The listing builds one solid part. Answer for the finished solid, in the listing's coordinates (mm). Coordinates: 2 decimals unless noted, no trailing zeros. Write each loop counter-clockwise with the first axis right and the second up, starting at its lowest first coordinate (ties: lowest second). Pieces come first, ordered by that corner, then holes.
from build123d import *

# Parameters (mm, degrees)
EXTRUDE_1_DEPTH     = 2
SKETCH_2_R          = 7.5
CUT_EXTRUDE_1_DEPTH = 52.974352649
SKETCH_3_R          = 2.5
CUT_EXTRUDE_2_DEPTH = 52.974352649
FILLET_2_R          = 5
SKETCH_4_R          = 1.5
CUT_EXTRUDE_3_DEPTH = 3


with BuildPart() as part:
    # 草图1 → 凸台-拉伸1 (new body)
    with BuildSketch(Plane.XY):
        Polygon((39.259818305, 0), (-19.629909152, 34), (-19.629909152, -34), align=None)
    extrude(amount=EXTRUDE_1_DEPTH)

    # 草图2 → 切除-拉伸1 (cut, through all)
    with BuildSketch(Plane.XY.offset(2)):
        Circle(SKETCH_2_R)
    extrude(amount=-CUT_EXTRUDE_1_DEPTH, mode=Mode.SUBTRACT)

    # 草图3 → 切除-拉伸2 (cut, through all)
    with BuildSketch(Plane.XY.offset(2)):
        with Locations((29, 0)):
            Circle(SKETCH_3_R)
        with Locations((-14.5, -25.11473671)):
            Circle(SKETCH_3_R)
        with Locations((-14.5, 25.11473671)):
            Circle(SKETCH_3_R)
    extrude(amount=-CUT_EXTRUDE_2_DEPTH, mode=Mode.SUBTRACT)

    # 圆角2
    fillet_2_edges = [part.edges().sort_by_distance(p)[0] for p in [
        (-19.629909152, -34, 1),
        (-19.629909152, 34, 1),
        (39.259818305, 0, 1),
    ]]
    fillet(fillet_2_edges, radius=FILLET_2_R)

    # 草图4 → 切除-拉伸3 (cut)
    with BuildSketch(Plane(origin=(0, 0, 0), x_dir=(-1, 0, 0), z_dir=(0, 0, -1))):
        with Locations(Location((-3.533865663, -13.120834875, 0), (0, 0, 180))):
            Circle(SKETCH_4_R)
        with Locations((-9.596043489, -9.620834875)):
            Circle(SKETCH_4_R)
    extrude(amount=-CUT_EXTRUDE_3_DEPTH, mode=Mode.SUBTRACT)


solid = part.part
Q1. The part is cut by section A-A, the plane y = 0. Write down the section's boundary in (x, z).
Answers below:
outline: (-19.63, 0) - (-7.5, 0) - (-7.5, 2) - (-19.63, 2) - close; (7.5, 0) - (26.5, 0) - (26.5, 2) - (7.5, 2) - close; (31.5, 0) - (34.26, 0) - (34.26, 2) - (31.5, 2) - close
Q2. The part is cut by section C-C, the plane x = 0. Write down the section's boundary in (y, z), then the cut area to 3 significant figures.
Answers below:
outline: (-22.67, 0) - (-7.5, 0) - (-7.5, 2) - (-22.67, 2) - close; (7.5, 0) - (22.67, 0) - (22.67, 2) - (7.5, 2) - close
area: 60.7 mm2
Q3. Find the intervals of material crossed by probe 1 along Y at (x, z) = (-14.5, 1.5); probe 2 along Y at (x, z) = (4, 1.45); probe 3 along Y at (x, z) = (0, 0.9), in increasing order.
Answers below:
probe 1: y = -30.34 to -27.61, -22.61 to 22.61, 27.61 to 30.34
probe 2: y = -20.36 to -14.55, -11.7 to -6.34, 6.34 to 20.36
probe 3: y = -22.67 to -7.5, 7.5 to 22.67
Q4. The part is cut by section B-B, the plane x = -14.5. Write down the section's boundary in (y, z), then the cut area to 3 significant figures.
Answers below:
outline: (-30.34, 0) - (-27.61, 0) - (-27.61, 2) - (-30.34, 2) - close; (-22.61, 0) - (22.61, 0) - (22.61, 2) - (-22.61, 2) - close; (27.61, 0) - (30.34, 0) - (30.34, 2) - (27.61, 2) - close
area: 101 mm2
Q5. The part is cut by section D-D, the plane z = 1.7. Write down the section's boundary in (x, y).
Answers below:
outline: (-19.63, -25.34) arc R5 ccw to (-12.13, -29.67) - (31.76, -4.33) arc R5 ccw to (31.76, 4.33) - (-12.13, 29.67) arc R5 ccw to (-19.63, 25.34) - close; hole circle Ø5 at (-14.5, -25.11); hole circle Ø5 at (-14.5, 25.11); hole circle Ø15 at (0, 0); hole circle Ø3 at (3.53, -13.12); hole circle Ø3 at (9.6, -9.62); hole circle Ø5 at (29, 0)
Q6. Given pin 1 (4.5 mm diameter, centred on x = 29, y = 0, fed in from +Z), flat-ended and moving along its own axis, determine where the tip first touches the part or whether it passes through.
Answers below:
pin 1: passes through
Q7. Determine the mould class of faces 1 (the face through (-14.825, -22.636, 1.014)), 2 (the face through (-5, 7, 2)), 3 (the face through (-19.63, 0, 1)) for opening direction X: released by +X, released by -X, zero draft, split by the parting line, or undercut.
Answers below:
face 1: undercut
face 2: zero draft
face 3: released by -X
